from build123d import *

# Parameters (mm, degrees)
SKETCH1_W               = 80
SKETCH1_H               = 45.4
SKETCH1_R               = 1.65
BOSS_EXTRUDE1_DEPTH     = 10.5
SKETCH2_W               = 5
SKETCH2_H               = 45.4
BOSS_EXTRUDE2_DEPTH     = 10.5
CUT_EXTRUDE1_DEPTH      = 7.8
CUT_EXTRUDE1_DEPTH_BACK = 93.58190968
SKETCH3_W               = 80
SKETCH3_H               = 12.2
SKETCH4_W               = 30
SKETCH4_H               = 8
BOSS_EXTRUDE3_DEPTH     = 44.2
SKETCH5_R               = 12
CUT_EXTRUDE2_DEPTH      = 45
CUT_EXTRUDE3_DEPTH      = 96.828388278
CUT_EXTRUDE3_DEPTH_BACK = 96.828388278
SKETCH6_R               = 2.6
FILLET1_SIZE            = 6
FILLET1_SIZE_2          = 15
SKETCH8_R               = 3.35
CUT_EXTRUDE5_DEPTH      = 8.5
SKETCH12_W              = 45
SKETCH12_H              = 12.25
CUT_EXTRUDE8_DEPTH      = 8.5
SKETCH13_W              = 14
SKETCH13_H              = 23.274164218
CUT_EXTRUDE10_DEPTH     = 10
SKETCH15_R              = 2.75
BOSS_EXTRUDE6_DEPTH     = 2
SKETCH16_W              = 43.180372268
SKETCH16_H              = 10.5
CUT_EXTRUDE11_DEPTH     = 12.5
CHAMFER2_SIZE2          = 12.5
CHAMFER2_SIZE           = 4.549627928
SKETCH17_R              = 2.2
CUT_EXTRUDE12_DEPTH     = 10
CUT_EXTRUDE13_DEPTH     = 102.559280367
SKETCH19_W              = 5
SKETCH19_H              = 24.2
BOSS_EXTRUDE7_DEPTH     = 5
SKETCH20_W              = 1
SKETCH20_H              = 12.2
CUT_EXTRUDE14_DEPTH     = 102.559280367
SKETCH21_W              = 5
SKETCH21_H              = 9.5
BOSS_EXTRUDE8_DEPTH     = 12.2
FILLET2_R               = 1
FILLET3_R               = 13
CHAMFER1_SIZE           = 2
SKETCH22_W              = 38.63074434
SKETCH22_H              = 1
BOSS_EXTRUDE9_DEPTH     = 3
SKETCH23_W              = 38.4
SKETCH23_H              = 1
BOSS_EXTRUDE10_DEPTH    = 3
CHAMFER3_SIZE           = 3


# Some blends are built 0.0001 mm under size
with BuildPart() as part:
    # Sketch1 → Boss-Extrude1 (new body)
    with BuildSketch(Plane.XY):
        with Locations((40, 22.7)):
            Rectangle(SKETCH1_W, SKETCH1_H)
        with Locations(Location((8.499989197, 32.7, 0), (0, 0, 180))):
            Circle(SKETCH1_R, mode=Mode.SUBTRACT)
        with Locations(Location((28.499989197, 32.7, 0), (0, 0, 180))):
            Circle(SKETCH1_R, mode=Mode.SUBTRACT)
        with Locations(Location((28.499989197, 12.7, 0), (0, 0, 180))):
            Circle(SKETCH1_R, mode=Mode.SUBTRACT)
        with Locations(Location((8.499989197, 12.7, 0), (0, 0, 180))):
            Circle(SKETCH1_R, mode=Mode.SUBTRACT)
    extrude(amount=BOSS_EXTRUDE1_DEPTH)

    # Sketch2 → Boss-Extrude2 (add)
    with BuildSketch(Plane(origin=(0, 0, 0), x_dir=(-1, 0, 0), z_dir=(0, 0, -1))):
        with Locations((-2.5, 22.7)):
            Rectangle(SKETCH2_W, SKETCH2_H)
    extrude(amount=BOSS_EXTRUDE2_DEPTH)

    # Sketch3 → Cut-Extrude1 (cut, two sides: drawn at the far end of the back side and taken through both)
    with BuildSketch(Plane.XY.offset(-CUT_EXTRUDE1_DEPTH_BACK)):
        with Locations((40, 22.7)):
            Rectangle(SKETCH3_W, SKETCH3_H)
    extrude(amount=CUT_EXTRUDE1_DEPTH + CUT_EXTRUDE1_DEPTH_BACK, mode=Mode.SUBTRACT)

    # Sketch4 → Boss-Extrude3 (add)
    with BuildSketch(Plane(origin=(0, 0, 0), x_dir=(-1, 0, 0), z_dir=(0, 0, -1))):
        with Locations((-54.5, 4)):
            Rectangle(SKETCH4_W, SKETCH4_H)
    extrude(amount=BOSS_EXTRUDE3_DEPTH)

    # Sketch5 → Cut-Extrude2 (cut)
    with BuildSketch(Plane(origin=(0, 8, 0), x_dir=(1, 0, 0), z_dir=(0, 1, 0))):
        with Locations(Location((54.495569327, 23.5, 0), (0, 0, 270))):
            Circle(SKETCH5_R)
    extrude(amount=-CUT_EXTRUDE2_DEPTH, mode=Mode.SUBTRACT)

    # Sketch6 → Cut-Extrude3 (cut, two sides: drawn at the far end of the back side and taken through both)
    with BuildSketch(Plane.XZ.offset(-16.6).offset(-CUT_EXTRUDE3_DEPTH_BACK)):
        with Locations((54.495569327, -39.201340103)):
            Circle(SKETCH6_R)
        with Locations((65.809277826, -34.515048602)):
            Circle(SKETCH6_R)
        with Locations((43.181860828, -34.515048602)):
            Circle(SKETCH6_R)
        with Locations((43.181860828, -11.887631605)):
            Circle(SKETCH6_R)
        with Locations((65.809277826, -11.887631605)):
            Circle(SKETCH6_R)
    extrude(amount=CUT_EXTRUDE3_DEPTH + CUT_EXTRUDE3_DEPTH_BACK, mode=Mode.SUBTRACT)

    # Fillet1
    # a fillet whose section is not a circle: 15, 6 mm, written as the material it takes off along each edge
    with BuildSketch(Plane(origin=(39.5, -37.5, -44.2), x_dir=(0, 0, 1), z_dir=(0, 1, 0)), Plane(origin=(69.5, 45.5, -44.2), x_dir=(0, 0, 1), z_dir=(0, -1, 0))) as fillet1_piece_1:
        with BuildLine():
            Bezier((FILLET1_SIZE, 0), (0, 0), (0, FILLET1_SIZE_2), weights=[1, 0.428571429, 1])
            Line((0, FILLET1_SIZE_2), (0, 0))
            Line((0, 0), (FILLET1_SIZE, 0))
        make_face()
    extrude(amount=83, mode=Mode.SUBTRACT)

    # Sketch8 → Cut-Extrude5 (cut)
    with BuildSketch(Plane.XY.offset(10.5)):
        with Locations((8.499989197, 32.7)):
            Circle(SKETCH8_R)
        with Locations((28.499989197, 32.7)):
            Circle(SKETCH8_R)
        with Locations((8.499989197, 12.7)):
            Circle(SKETCH8_R)
        with Locations((28.499989197, 12.7)):
            Circle(SKETCH8_R)
    extrude(amount=-CUT_EXTRUDE5_DEPTH, mode=Mode.SUBTRACT)

    # Sketch12 → Cut-Extrude8 (cut)
    with BuildSketch(Plane.XY.offset(10.5)):
        with Locations((22.5, 39.275)):
            Rectangle(SKETCH12_W, SKETCH12_H)
    extrude(amount=-CUT_EXTRUDE8_DEPTH, mode=Mode.SUBTRACT)

    # Sketch13 → Cut-Extrude10 (cut)
    with BuildSketch(Plane(origin=(0, 8, 0), x_dir=(1, 0, 0), z_dir=(0, 1, 0))):
        with Locations((54.495569327, 39.201340103)):
            Rectangle(SKETCH13_W, SKETCH13_H)
    extrude(amount=-CUT_EXTRUDE10_DEPTH, mode=Mode.SUBTRACT)

    # Sketch15 → Boss-Extrude6 (add)
    with BuildSketch(Plane(origin=(0, 8, 0), x_dir=(1, 0, 0), z_dir=(0, 1, 0))):
        with Locations(Location((54.495569327, 7.201340104, 0), (0, 0, 90))):
            Circle(SKETCH15_R)
    extrude(amount=BOSS_EXTRUDE6_DEPTH)

    # Sketch16 → Cut-Extrude11 (cut)
    with BuildSketch(Plane(origin=(0, 45.4, 0), x_dir=(1, 0, 0), z_dir=(0, 1, 0))):
        with Locations((53.409813866, -5.25)):
            Rectangle(SKETCH16_W, SKETCH16_H)
    extrude(amount=-CUT_EXTRUDE11_DEPTH, mode=Mode.SUBTRACT)

    # Chamfer2
    chamfer2_edges = [part.edges().sort_by_distance(p)[0] for p in [
        (75, 32.9, 5.25),
    ]]
    chamfer2_side = [part.faces().sort_by_distance(p)[0] for p in [
        (74.909007441, 32.9, 5.25),
    ]]
    chamfer(chamfer2_edges, length=CHAMFER2_SIZE - 0.0001, length2=CHAMFER2_SIZE2 - 0.0001, reference=chamfer2_side[0])  # a hair under: the kernel refuses the full size

    # Sketch17 → Cut-Extrude12 (cut)
    with BuildSketch(Plane(origin=(80, 0, 0), x_dir=(0, 0, -1), z_dir=(1, 0, 0))):
        with Locations((-5.3, 39.15)):
            Circle(SKETCH17_R)
    extrude(amount=-CUT_EXTRUDE12_DEPTH, mode=Mode.SUBTRACT)

    # Sketch18 → Cut-Extrude13 (cut, through all)
    with BuildSketch(Plane(origin=(80, 0, 0), x_dir=(0, 0, -1), z_dir=(1, 0, 0))):
        Polygon((-7.8, 28.8), (-6.8, 28.8), (-7.8, 29.3), align=None)
        Polygon((-7.8, 16.6), (-7.8, 16.1), (-6.8, 16.6), align=None)
    extrude(amount=-CUT_EXTRUDE13_DEPTH, mode=Mode.SUBTRACT)

    # Sketch19 → Boss-Extrude7 (add)
    with BuildSketch(Plane(origin=(0, 0, 0), x_dir=(-1, 0, 0), z_dir=(0, 0, -1))):
        with Locations((-77.5, 22.7)):
            Rectangle(SKETCH19_W, SKETCH19_H)
    extrude(amount=BOSS_EXTRUDE7_DEPTH)

    # Sketch20 → Cut-Extrude14 (cut, through all)
    with BuildSketch(Plane(origin=(80, 0, 0), x_dir=(0, 0, -1), z_dir=(1, 0, 0))):
        with Locations((0.5, 22.7)):
            Rectangle(SKETCH20_W, SKETCH20_H)
    extrude(amount=-CUT_EXTRUDE14_DEPTH, mode=Mode.SUBTRACT)

    # Sketch21 → Boss-Extrude8 (add)
    with BuildSketch(Plane(origin=(0, 16.6, 0), x_dir=(1, 0, 0), z_dir=(0, 1, 0))):
        with Locations((2.5, 5.75)):
            Rectangle(SKETCH21_W, SKETCH21_H)
    extrude(amount=BOSS_EXTRUDE8_DEPTH)

    # Fillet2
    fillet2_edges = [part.edges().sort_by_distance(p)[0] for p in [
        (77.5, 16.6, -1),
        (77.5, 28.8, -1),
        (2.5, 16.6, -1),
        (2.5, 28.8, -1),
    ]]
    fillet(fillet2_edges, radius=FILLET2_R)

    # Fillet3
    # the kernel refuses this fillet: 13 mm, written as the material it adds along each edge
    with BuildSketch(Plane(origin=(80, 10.6, 0), x_dir=(0, -1, 0), z_dir=(-1, 0, 0)), Plane(origin=(75, 34.8, 0), x_dir=(0, 1, 0), z_dir=(1, 0, 0))) as fillet3_piece_1:
        with BuildLine():
            CenterArc((10.246950766, -13), FILLET3_R, 90, 52.020127555)
            Line((0, -5), (0, 0))
            Line((0, 0), (10.246950766, 0))
        make_face()
    extrude(amount=5)

    # Chamfer1
    chamfer1_edges = [part.edges().sort_by_distance(p)[0] for p in [
        (54.495569327, 10, -4.451340104),
    ]]
    chamfer(chamfer1_edges, length=CHAMFER1_SIZE - 0.0001)  # a hair under: the kernel refuses the full size

    # Sketch22 → Boss-Extrude9 (add)
    with BuildSketch(Plane.XY.offset(10.5)):
        with Locations((51.134999902, 32.4)):
            Rectangle(SKETCH22_W, SKETCH22_H)
    extrude(amount=BOSS_EXTRUDE9_DEPTH)

    # Sketch23 → Boss-Extrude10 (add)
    with BuildSketch(Plane(origin=(0, 0, 0), x_dir=(-1, 0, 0), z_dir=(0, 0, -1))):
        with Locations((-51.250372072, 32.4)):
            Rectangle(SKETCH23_W, SKETCH23_H)
    extrude(amount=BOSS_EXTRUDE10_DEPTH)

    # Chamfer3
    chamfer3_edges = [part.edges().sort_by_distance(p)[0] for p in [
        (51.134999902, 31.9, 10.5),
        (51.250372072, 31.9, 0),
    ]]
    chamfer(chamfer3_edges, length=CHAMFER3_SIZE - 0.0001)  # a hair under: the kernel refuses the full size


solid = part.part
Verification items for the finished model (mm, model axes). A direction names the side the tool comes from. Coordinates: 2 decimals unless noted, no trailing zeros. Order: outer loops, then holes, each group sorted by start corner. A loop starts at its lowest first (then second) coordinate and runs counter-clockwise, first axis right, second up. Notation, with made-up numbers: M 51.25,21.25 L 91.25,21.25 A10 cw 91.25,26.25 Z; hole C 45.25,-36.75 d10. An arc over 180 degrees is marked long. Return JSON: item names as keys, results as strings.
1) Cross-section at B-B, the plane z = 5. Count the separate pieces of the cut face and the enclosed holes in it, and give its area (3 significant figures).
Answer list:
{"separate pieces": "3", "enclosed holes": "2", "area": "1,610 mm2"}
2) Release check for a two-part mould opening along X. For faces 1 (the flat face through (80, 22, 8)), 2 (the flat face through (49, 0, -4)), 3 (the cylindrical face through (25.842, 10.662, 6.31)) record: +X half, -X half, draft (parallel to the pull), parting line (faces both ways), or undercut.
Answer list:
{"face 1": "+X half", "face 2": "draft", "face 3": "undercut"}
3) Cross-section at C-C, the plane z = -28. Record the boundary of the cut face in (x, y).
Answer list:
{"outline": "M 39.5,0 L 43.37,0 L 43.37,8 L 39.5,8 Z; M 65.62,0 L 69.5,0 L 69.5,8 L 65.62,8 Z"}
4) Access from +Z, -Z, +X, -X, +Y, -Y to the whole of each face (thin tool, end or side, straight path). Record for faces 4 (the flat face through (51.5, 30.4, -1.5)), 5 (the flat face through (51, 32.9, 5)), 6 (the flat face through (2, 22, -10.5)).
Answer list:
{"face 4": "-Z", "face 5": "+Z, -Z, +Y", "face 6": "-Z, -X, +Y, -Y"}
5) Cross-section at A-A, the plane y = 12.7. Record the boundary of the cut face in (x, z), and give its area (3 significant figures).
Answer list:
{"outline": "M 0,-10.5 L 5,-10.5 L 5,0 L 6.85,0 L 6.85,2 L 5.15,2 L 5.15,10.5 L 0,10.5 Z; M 10.15,0 L 26.85,0 L 26.85,2 L 25.15,2 L 25.15,10.5 L 11.85,10.5 L 11.85,2 L 10.15,2 Z; M 30.15,0 L 75,0 L 75,-5 L 80,-5 L 80,10.5 L 31.85,10.5 L 31.85,2 L 30.15,2 Z", "area": "790 mm2"}
6) Gauge pin test, flat ends, axial feed: pin 1 (3 mm diameter, centred on x = 21.5, y = 37, fed in from +Z); pin 2 (8.5 mm diameter, centred on x = 27, y = 39.5, fed in from -Z); pin 3 (2.5 mm diameter, centred on y = 2.5, z = -37.5, fed in from -X). Record the tip position at first contact, or that the pin passes through.
Answer list:
{"pin 1": "z = 2", "pin 2": "z = 0", "pin 3": "x = 39.5"}
7) Thickness scan on L1, parallel to X at y = 32.7, z = 0.65; L2, parallel to X at y = 12, z = 5; L3, parallel to Z at x = 26.5, y = 33. Record the ranges inside material, lowest first. Write a range as [from, to].
Answer list:
{"L1": "[0, 6.85], [10.15, 26.85], [30.15, 80]", "L2": "[0, 5.22], [11.78, 25.22], [31.78, 80]", "L3": "[0, 2]"}
8) Cross-section at D-D, the plane x = 74. Record the boundary of the cut face in (y, z), and give its area (3 significant figures).
Answer list:
{"outline": "M 0,0 L 16.6,0 L 16.6,6.8 L 16.1,7.8 L 29.3,7.8 L 28.8,6.8 L 28.8,0 L 42.65,0 L 42.65,10.5 L 0,10.5 Z; hole C 39.15,5.3 d4.4", "area": "337 mm2"}
